The listing builds one solid part. Answer for the finished solid, in the listing's coordinates (mm). Give positions to 0.01 mm unless a question says otherwise; leave off trailing zeros. Write each loop counter-clockwise with the first axis right and the second up, starting at its lowest first coordinate (ties: lowest second). Pieces come first, ordered by that corner, then holes. Notation, with made-up numbers: (81.25, -38.75) - (90.25, -38.75) arc R26 ccw to (90.25, -4.75) - close; hole circle Ø1 at (-24, -23). An arc over 180 degrees is marked (long way). Answer in a Markdown table with one row per item. Add a question column.
from build123d import *

# Parameters (mm, degrees)
SKETCH_1_W          = 26.5
SKETCH_1_H          = 50
EXTRUDE_1_DEPTH     = 4
SKETCH_2_R          = 1.525
CUT_EXTRUDE_1_DEPTH = 4
FILLET_1_R          = 3


with BuildPart() as part:
    # 草图1 → 凸台-拉伸1 (new body)
    with BuildSketch(Plane.XY):
        Rectangle(SKETCH_1_W, SKETCH_1_H)
    extrude(amount=EXTRUDE_1_DEPTH)

    # 草图2 → 切除-拉伸1 (cut)
    with BuildSketch(Plane.XY.offset(4)):
        with Locations((-10.158640444, 9)):
            Circle(SKETCH_2_R)
        with Locations((1.841359556, 9)):
            Circle(SKETCH_2_R)
        with Locations((-10.158640444, -11)):
            Circle(SKETCH_2_R)
        with Locations((1.841359556, -11)):
            Circle(SKETCH_2_R)
    extrude(amount=-CUT_EXTRUDE_1_DEPTH, mode=Mode.SUBTRACT)

    # 圆角1
    fillet_1_edges = [part.edges().sort_by_distance(p)[0] for p in [
        (13.25, -25, 2),
        (-13.25, -25, 2),
        (-13.25, 25, 2),
        (13.25, 25, 2),
    ]]
    fillet(fillet_1_edges, radius=FILLET_1_R)


solid = part.part
1. Straight lines are drawn through the part: L1, parallel to Y at x = 1.25, z = 3.4; L2, parallel to Y at x = -11.5, z = 1.7; L3, parallel to Y at x = -12, z = 2.9. For each, find the intervals that lie inside material, in ascending order. Write a range as [from, to].
2. Section B-B (z = 1.8) is taken. Give the vertices of the cut face in (x, y) (3 decimals).
3. Section C-C (y = -12) is taken. Give the vertices of the cut face in (x, z), and give its area (3 significant figures).
4. Section A-A (y = 9) is taken. Give the vertices of the cut face in (x, z).
5. Given pin 1 Ø3 at (x, y) = (-4, -5) entering from -Z; pin 2 Ø2.5 at (x, y) = (1.84, -11) entering from -Z, each flat-ended and moving along its own axis, determine where each tip first touches the part or whether it passes through.
Geometry check:
| question | item | result |
|---|---|---|
| 1 | L1 | [-25, -12.41], [-9.59, 7.59], [10.41, 25] |
| 1 | L2 | [-24.73, -11.73], [-10.27, 8.27], [9.73, 24.73] |
| 1 | L3 | [-24.44, 24.44] |
| 2 | outline | (-13.25, -22) arc R3 ccw to (-10.25, -25) - (10.25, -25) arc R3 ccw to (13.25, -22) - (13.25, 22) arc R3 ccw to (10.25, 25) - (-10.25, 25) arc R3 ccw to (-13.25, 22) - close; hole circle Ø3.05 at (-10.159, -11); hole circle Ø3.05 at (-10.159, 9); hole circle Ø3.05 at (1.841, -11); hole circle Ø3.05 at (1.841, 9) |
| 3 | outline | (-13.25, 0) - (-11.31, 0) - (-11.31, 4) - (-13.25, 4) - close; (-9.01, 0) - (0.69, 0) - (0.69, 4) - (-9.01, 4) - close; (2.99, 0) - (13.25, 0) - (13.25, 4) - (2.99, 4) - close |
| 3 | area | 87.6 mm² |
| 4 | outline | (-13.25, 0) - (-11.68, 0) - (-11.68, 4) - (-13.25, 4) - close; (-8.63, 0) - (0.32, 0) - (0.32, 4) - (-8.63, 4) - close; (3.37, 0) - (13.25, 0) - (13.25, 4) - (3.37, 4) - close |
| 5 | pin 1 | z = 0 |
| 5 | pin 2 | through |
